from build123d import *

# Parameters (mm, degrees)
BOSS_EXTRUDE1_START     = -3
BOSS_EXTRUDE1_OUTLINE_W = 2.8
BOSS_EXTRUDE1_OUTLINE_H = 20
BOSS_EXTRUDE1_DEPTH     = 3
SKETCH2_W               = 3
SKETCH2_H               = 20
BOSS_EXTRUDE2_DEPTH     = 3
SKETCH3_W               = 20
SKETCH3_H               = 3
BOSS_EXTRUDE3_DEPTH     = 3
FILLET1_R               = 5
FILLET2_R               = 5


with BuildPart() as part:
    # Boss-Extrude1: read off the stored shape, not the designer's step
    # Boss-Extrude1 outline → Boss-Extrude1 (new body)
    with BuildSketch(Plane(origin=(3, 0, 0), x_dir=(0, 0, -1), z_dir=(1, 0, 0)).offset(BOSS_EXTRUDE1_START)):
        Polygon((55, 65), (55, 75), (-120, 95), (-120, 265), (-150, 265), (-150, 5), (-120, 5), (-120, 50), (40, 50), align=None)
        with Locations((-111.4, 67)):
            Rectangle(BOSS_EXTRUDE1_OUTLINE_W, BOSS_EXTRUDE1_OUTLINE_H, mode=Mode.SUBTRACT)
        with Locations((-101.4, 67)):
            Rectangle(BOSS_EXTRUDE1_OUTLINE_W, BOSS_EXTRUDE1_OUTLINE_H, mode=Mode.SUBTRACT)
        with Locations((8.6, 67)):
            Rectangle(BOSS_EXTRUDE1_OUTLINE_W, BOSS_EXTRUDE1_OUTLINE_H, mode=Mode.SUBTRACT)
        with Locations((18.6, 67)):
            Rectangle(BOSS_EXTRUDE1_OUTLINE_W, BOSS_EXTRUDE1_OUTLINE_H, mode=Mode.SUBTRACT)
        with Locations((-140, 215)):
            Rectangle(BOSS_EXTRUDE1_OUTLINE_W, BOSS_EXTRUDE1_OUTLINE_H, mode=Mode.SUBTRACT)
    extrude(amount=BOSS_EXTRUDE1_DEPTH)

    # Sketch2 → Boss-Extrude2 (add)
    with BuildSketch(Plane(origin=(0, 265, 0), x_dir=(1, 0, 0), z_dir=(0, 1, 0))):
        with Locations((1.5, -135)):
            Rectangle(SKETCH2_W, SKETCH2_H)
    extrude(amount=BOSS_EXTRUDE2_DEPTH)

    # Sketch3 → Boss-Extrude3 (add)
    with BuildSketch(Plane(origin=(3, 0, 0), x_dir=(0, 0, -1), z_dir=(1, 0, 0))):
        with Locations((-135, 3.5)):
            Rectangle(SKETCH3_W, SKETCH3_H)
        Polygon((40, 50), (40, 5), (35, 5), (35, 2), (15, 2), (15, 5), (10, 5), (10, 50), align=None)
    extrude(amount=-BOSS_EXTRUDE3_DEPTH)

    # Fillet1
    fillet1_edges = [part.edges().sort_by_distance(p)[0] for p in [
        (1.5, 65, -55),
        (1.5, 50, -10),
        (1.5, 75, -55),
        (1.5, 50, -40),
        (1.5, 50, 120),
    ]]
    fillet(fillet1_edges, radius=FILLET1_R)

    # Fillet2
    fillet2_edges = [part.edges().sort_by_distance(p)[0] for p in [
        (1.5, 95, 120),
    ]]
    fillet(fillet2_edges, radius=FILLET2_R)


solid = part.part
Can you work these out from the model? Positions are in its coordinate system, mm. Round coordinates to 2 decimals unless told otherwise and drop trailing zeros. Loops run counter-clockwise (first coordinate to the right, second up) from the corner with the lowest first, then second, coordinate; pieces in that order, holes last. Notation, with made-up numbers: (-31, 85.25) - (27, 85.25) arc R29 cw to (27, 115.25) - close; hole circle Ø9 at (61, -12.75). An arc over 180 degrees is marked (long way). Use CSV: the item, a comma, the result in double quotes. Start each with the question number.
1) If we section it at C-C on z = 57: Write out the boundary of the cut face in (x, y).
2) For pin 1 Ø1.4 at (x, z) = (1, -18.5) entering from +Y; pin 2 Ø1 at (x, z) = (0.5, 122) entering from +Y; pin 3 Ø1.5 at (x, z) = (2.5, 19.5) entering from -Y, each with a flat end and sliding along its axis, tell me the tip position at first contact or that it passes through.
3) If we section it at A-A on x = 2.5: Count the separate pieces of the cut face and the enclosed holes in it, plus the area to 3 significant figures.
4) Please list where these lines run through material, in increasing order: probe 1 along Z at (x, y) = (1.45, 68); probe 2 along Z at (x, y) = (1.5, 32); probe 3 along Z at (x, y) = (2.95, 196). Write a range as [from, to].
5) If we section it at B-B on y = 123: Write out the boundary of the cut face in (x, z), plus the area to 3 significant figures.
Geometry results:
1,outline,"(0, 50) - (3, 50) - (3, 87.8) - (0, 87.8) - close"
2,pin 1,"stops at y = 79.25"
2,pin 2,"stops at y = 265"
2,pin 3,"stops at y = 50"
3,separate pieces,"1"
3,enclosed holes,"5"
3,area,"15,100 mm2"
4,probe 1,"z = [-55, -20], [-17.2, -10], [-7.2, 100], [102.8, 110], [112.8, 150]"
4,probe 2,"z = [-40, -10], [120, 150]"
4,probe 3,"z = [120, 150]"
5,outline,"(0, 120) - (3, 120) - (3, 150) - (0, 150) - close"
5,area,"90.0 mm2"
